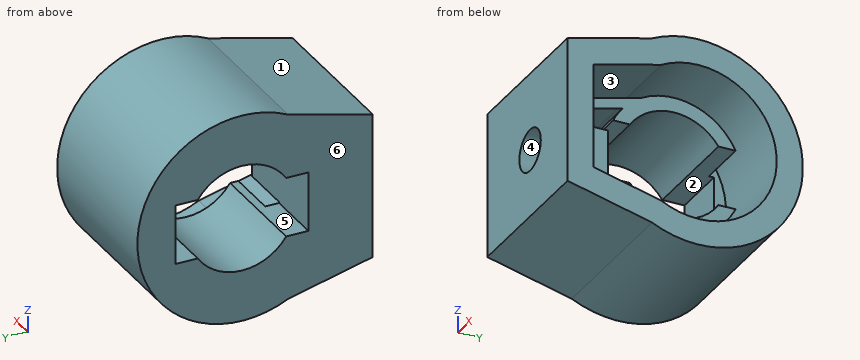
from build123d import *

# Parameters (mm, degrees)
CROQUIS1_R              = 10
SALIENTE_EXTRUIR1_DEPTH = 11
CROQUIS2_R              = 10
SALIENTE_EXTRUIR2_DEPTH = 10
CORTAR_EXTRUIR3_DEPTH   = 10
CROQUIS8_R              = 1.55
CORTAR_EXTRUIR4_DEPTH   = 5
CORTAR_EXTRUIR5_REACH   = 52.656
CORTAR_EXTRUIR6_START   = -10
CORTAR_EXTRUIR6_DEPTH   = 10
SALIENTE_EXTRUIR3_DEPTH = 30
CORTAR_EXTRUIR7_REACH   = 66.42
CROQUIS14_R             = 4


with BuildPart() as part:
    # Croquis1 → Saliente-Extruir1 (new body)
    with BuildSketch(Plane(origin=(0, 0, 0), x_dir=(0, 0, -1), z_dir=(1, 0, 0))):
        with BuildLine():
            Line((-5.780776406, 0), (-24.219223594, 0))
            Line((-24.219223594, 0), (-25, 0))
            Line((-25, 0), (-25.189366094, 0.757464375))
            Line((-25.189366094, 0.757464375), (-28.235294118, 12.941176471))
            ThreePointArc((-28.235294118, 12.941176471), (-15, 35), (-1.764705882, 12.941176471))
            Line((-1.764705882, 12.941176471), (-4.810633906, 0.757464375))
            Line((-4.810633906, 0.757464375), (-5, 0))
            Line((-5, 0), (-5.780776406, 0))
        make_face()
        with Locations((-15, 20)):
            Circle(CROQUIS1_R, mode=Mode.SUBTRACT)
    extrude(amount=SALIENTE_EXTRUIR1_DEPTH)

    # Croquis2 → Saliente-Extruir2 (add)
    with BuildSketch(Plane(origin=(11, 0, 0), x_dir=(0, 0, -1), z_dir=(1, 0, 0))):
        with BuildLine():
            Line((-23.477486008, 1.95), (-6.522513992, 1.95))
            Line((-6.522513992, 1.95), (-3.59620246, 13.655246131))
            ThreePointArc((-3.59620246, 13.655246131), (-15, 33.05), (-26.40379754, 13.655246131))
            Line((-26.40379754, 13.655246131), (-23.477486008, 1.95))
        make_face()
        with Locations((-15, 20)):
            Circle(CROQUIS2_R, mode=Mode.SUBTRACT)
    extrude(amount=SALIENTE_EXTRUIR2_DEPTH)

    # Croquis3 → Cortar-Extruir3 (cut)
    with BuildSketch(Plane(origin=(21, 0, 0), x_dir=(0, 0, -1), z_dir=(1, 0, 0))):
        Polygon((-9.522513992, 1.95), (-9.522513992, 9.95), (-4.522513992, 9.95), (-6.522513992, 1.95), align=None)
        with BuildLine():
            Line((-23.477486008, 1.95), (-18.477486008, 1.95))
            Line((-18.477486008, 1.95), (-18.477486008, 6.945227656))
            Line((-18.477486008, 6.945227656), (-18.477486008, 7.473743933))
            ThreePointArc((-18.477486008, 7.473743933), (-21.115240601, 8.528128645), (-23.461002355, 10.130276643))
            Line((-23.461002355, 10.130276643), (-23.242071918, 9.254554893))
            Line((-23.242071918, 9.254554893), (-21.915933195, 3.95))
            Line((-21.915933195, 3.95), (-23.977486008, 3.95))
            Line((-23.977486008, 3.95), (-23.477486008, 1.95))
        make_face()
    extrude(amount=-CORTAR_EXTRUIR3_DEPTH, mode=Mode.SUBTRACT)

    # Croquis8 → Cortar-Extruir4 (cut)
    with BuildSketch(Plane.XZ.offset(-1.95)):
        with Locations(Location((16, 14, 0), (0, 0, 270))):
            Circle(CROQUIS8_R)
    extrude(amount=-CORTAR_EXTRUIR4_DEPTH, mode=Mode.SUBTRACT)

    # Cortar-Extruir5: up to this face of the body (flat: up to its plane)
    cortar_extruir5_end = Plane(part.part.faces().sort_by_distance((21, 32.643992611, 15))[0])
    # Croquis11 → Cortar-Extruir5 (cut, up to the picked face)
    with BuildSketch(Plane.ZY, mode=Mode.PRIVATE) as cortar_extruir5_sk1:
        with BuildLine():
            Line((20.7, 32.7), (9.3, 32.7))
            Line((9.3, 32.7), (9.3, 28.458723308))
            ThreePointArc((9.3, 28.458723308), (4.8, 20), (9.3, 11.541276692))
            Line((9.3, 11.541276692), (9.3, 7.3))
            Line((9.3, 7.3), (20.7, 7.3))
            Line((20.7, 7.3), (20.7, 11.541276692))
            ThreePointArc((20.7, 11.541276692), (25.2, 20), (20.7, 28.458723308))
            Line((20.7, 28.458723308), (20.7, 32.7))
        make_face()
    cortar_extruir5_tool1 = split(extrude(cortar_extruir5_sk1.sketch, amount=-CORTAR_EXTRUIR5_REACH, mode=Mode.PRIVATE), bisect_by=cortar_extruir5_end, keep=Keep.BOTH, mode=Mode.PRIVATE)
    add(cortar_extruir5_tool1.solids().sort_by(Axis((0, 20, 15), (1, 0, 0)))[0], mode=Mode.SUBTRACT)

    # Croquis12 → Cortar-Extruir6 (cut)
    with BuildSketch(Plane(origin=(21, 0, 0), x_dir=(0, 0, -1), z_dir=(1, 0, 0)).offset(CORTAR_EXTRUIR6_START)):
        with BuildLine():
            Line((-18.00208261, 32.7), (-11.99791739, 32.7))
            ThreePointArc((-11.99791739, 32.7), (-15, 33.05), (-18.00208261, 32.7))
        make_face()
    extrude(amount=CORTAR_EXTRUIR6_DEPTH, mode=Mode.SUBTRACT)

    # Croquis13 → Saliente-Extruir3 (add)
    with BuildSketch(Plane.ZY):
        with BuildLine():
            Line((1.096117968, -5), (28.903882032, -5))
            Line((28.903882032, -5), (32.947577878, 11.174783385))
            ThreePointArc((32.947577878, 11.174783385), (15, 40), (-2.947577878, 11.174783385))
            Line((-2.947577878, 11.174783385), (1.096117968, -5))
        make_face()
        with BuildLine():
            Line((5, 0), (25, 0))
            Line((25, 0), (28.235294118, 12.941176471))
            ThreePointArc((28.235294118, 12.941176471), (15, 35), (1.764705882, 12.941176471))
            Line((1.764705882, 12.941176471), (5, 0))
        make_face(mode=Mode.SUBTRACT)
    extrude(amount=-SALIENTE_EXTRUIR3_DEPTH)

    # Croquis14 → Cortar-Extruir7 (cut, up to next)
    with BuildSketch(Plane.XZ.offset(5), mode=Mode.PRIVATE) as cortar_extruir7_sk1:
        with Locations(Location((16, 14, 0), (0, 0, 270))):
            Circle(CROQUIS14_R)
    cortar_extruir7_tool1 = extrude(cortar_extruir7_sk1.sketch, amount=-CORTAR_EXTRUIR7_REACH, mode=Mode.PRIVATE) & part.part
    add(cortar_extruir7_tool1.solids().sort_by_distance((16, -5, 14))[0], mode=Mode.SUBTRACT)


solid = part.part
Source: CAD feature listing. Evaluate the final solid. Frame: model axes, mm. Face numbers are marked on the shaded views. A direction names the side the tool comes from. Round coordinates to 2 decimals unless told otherwise and drop trailing zeros. Order: outer loops, then holes, each group sorted by start corner. A loop starts at its lowest first (then second) coordinate and runs counter-clockwise, first axis right, second up. Notation, with made-up numbers: (76.5, 4.5) -> (101.5, 4.5) arc R19 cw to (101.5, 40.5) -> close; hole circle Ø8 at (89.5, 14.5). An arc over 180 degrees is marked (long way). Answer as CSV lines item,"result".
Item 1: Pull-direction query (X, two-part tool) for the marked faces 4, 5 and 6; classes: pulls with the +X half, pulls with the -X half, needs draft (parallel to the pull), parting line crosses it, or undercut.
A:
face 4,"undercut"
face 5,"needs draft"
face 6,"pulls with the -X half"
Item 2: Section B-B, the plane y = 20. Return loops of the section in (x, z), plus the area to 3 significant figures.
A:
outline,"(0, -5) -> (30, -5) -> (30, 0) -> (11, 0) -> (11, 1.95) -> (21, 1.95) -> (21, 4.8) -> (0, 4.8) -> close; (0, 25.2) -> (21, 25.2) -> (21, 28.05) -> (11, 28.05) -> (11, 30) -> (30, 30) -> (30, 35) -> (0, 35) -> close"
area,"463 mm²"
Item 3: Section C-C, the plane z = 15. Return loops of the section in (x, y).
A:
outline,"(0, -5) -> (12.13, -5) -> (12.13, 0) -> (11, 0) -> (11, 1.95) -> (14.82, 1.95) -> (14.82, 6.95) -> (17.18, 6.95) -> (17.18, 1.95) -> (21, 1.95) -> (21, 7.3) -> (0, 7.3) -> close; (0, 32.7) -> (11, 32.7) -> (11, 35) -> (30, 35) -> (30, 40) -> (0, 40) -> close; (19.87, -5) -> (30, -5) -> (30, 0) -> (19.87, 0) -> close"
Item 4: Reachability of the marked faces 1, 2 and 3 from +Z, -Z, +X, -X, +Y, -Y: full face, straight path, thin tool, end or side. Return the list, or none.
A:
face 1,"+Z, +X, -X, -Y"
face 2,"+X, -X"
face 3,"+X"
Item 5: Line query: L1, parallel to X at y = 5.85, z = 14; L2, parallel to Y at x = 25.75, z = 15; L3, parallel to Y at x = 11.75, z = 16. Output: solid intervals per line, ascending.
A:
L1,"0 to 14.45, 17.55 to 21"
L2,"-5 to 0, 35 to 40"
L3,"-5 to 0, 1.95 to 7.3, 34.97 to 39.97"
Item 6: Section D-D, the plane y = -1.5. Return loops of the section in (x, z).
A:
outline,"(0, 0.22) -> (30, 0.22) -> (30, 29.78) -> (0, 29.78) -> close; hole circle Ø8 at (16, 14)"
Item 7: Pin query (flat end, axial travel): pin 1 Ø1 at (x, z) = (18, 21) entering from +Y; pin 2 Ø3.5 at (x, z) = (6, 17.5) entering from +Y; pin 3 Ø6.5 at (x, z) = (16, 14) entering from -Y; pin 4 Ø1 at (y, z) = (22, 24) entering from +X. Return the tip coordinate at first contact, or that it passes through.
A:
pin 1,"y = 39.23"
pin 2,"y = 39.99"
pin 3,"y = 1.95"
pin 4,"through"
Item 8: Section A-A, the plane x = 27. Return loops of the section in (y, z), plus the area to 3 significant figures.
A:
outline,"(-5, 1.1) -> (11.17, -2.95) arc R20 ccw (long way) to (11.17, 32.95) -> (-5, 28.9) -> close; hole (0, 5) -> (12.94, 1.76) arc R15 ccw (long way) to (12.94, 28.24) -> (0, 25) -> close"
area,"627 mm²"
